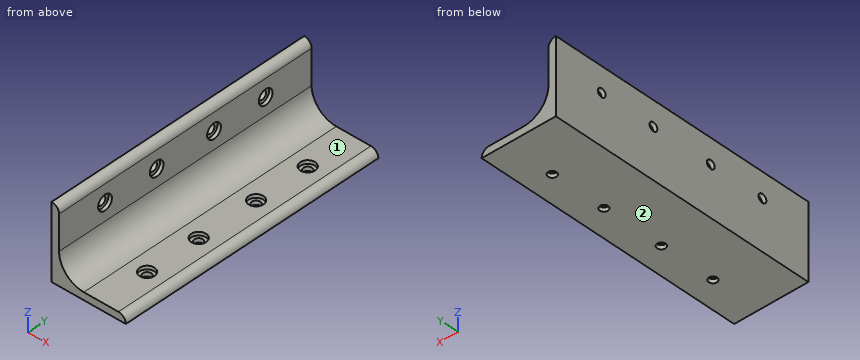
from build123d import *

# Parameters (mm, degrees)
BOSS_EXTRUDE1_DEPTH = 110
FILLET1_R           = 10
FILLET2_R           = 3
SKETCH2_R           = 1.7
CUT_EXTRUDE1_DEPTH  = 118.170815479
SKETCH3_R           = 1.7
CUT_EXTRUDE2_DEPTH  = 118.170815479
SKETCH4_R           = 3
CUT_EXTRUDE3_DEPTH  = 1.4
SKETCH5_R           = 3
CUT_EXTRUDE4_DEPTH  = 1.4


with BuildPart() as part:
    # Sketch1 → Boss-Extrude1 (new body)
    with BuildSketch(Plane(origin=(0, 0, 0), x_dir=(1, 0, 0), z_dir=(0, 1, 0))):
        Polygon((0, 0), (0, -30), (3, -30), (3, -3), (30, -3), (30, 0), align=None)
    extrude(amount=BOSS_EXTRUDE1_DEPTH)

    # Fillet1
    fillet1_edges = [part.edges().sort_by_distance(p)[0] for p in [
        (3, 55, 3),
    ]]
    fillet(fillet1_edges, radius=FILLET1_R)

    # Fillet2
    fillet2_edges = [part.edges().sort_by_distance(p)[0] for p in [
        (3, 55, 30),
        (30, 55, 3),
    ]]
    fillet(fillet2_edges, radius=FILLET2_R - 0.0001)  # a hair under: the kernel refuses the full size

    # Sketch2 → Cut-Extrude1 (cut, through all)
    with BuildSketch(Plane.XY.offset(3)):
        with Locations((20, 90)):
            Circle(SKETCH2_R)
        with Locations(Location((20, 67.5, 0), (0, 0, 180))):
            Circle(SKETCH2_R)
        with Locations((20, 42.5)):
            Circle(SKETCH2_R)
        with Locations(Location((20, 20, 0), (0, 0, 180))):
            Circle(SKETCH2_R)
    extrude(amount=-CUT_EXTRUDE1_DEPTH, mode=Mode.SUBTRACT)

    # Sketch3 → Cut-Extrude2 (cut, through all)
    with BuildSketch(Plane(origin=(3, 0, 0), x_dir=(0, 0, -1), z_dir=(1, 0, 0))):
        with Locations((-20, 90)):
            Circle(SKETCH3_R)
        with Locations(Location((-20, 67.5, 0), (0, 0, 180))):
            Circle(SKETCH3_R)
        with Locations((-20, 42.5)):
            Circle(SKETCH3_R)
        with Locations(Location((-20, 20, 0), (0, 0, 180))):
            Circle(SKETCH3_R)
    extrude(amount=-CUT_EXTRUDE2_DEPTH, mode=Mode.SUBTRACT)

    # Sketch4 → Cut-Extrude3 (cut)
    with BuildSketch(Plane.XY.offset(3)):
        with Locations((20, 90)):
            Circle(SKETCH4_R)
        with Locations(Location((20, 67.5, 0), (0, 0, 180))):
            Circle(SKETCH4_R)
        with Locations((20, 42.5)):
            Circle(SKETCH4_R)
        with Locations(Location((20, 20, 0), (0, 0, 180))):
            Circle(SKETCH4_R)
    extrude(amount=-CUT_EXTRUDE3_DEPTH, mode=Mode.SUBTRACT)

    # Sketch5 → Cut-Extrude4 (cut)
    with BuildSketch(Plane(origin=(3, 0, 0), x_dir=(0, 0, -1), z_dir=(1, 0, 0))):
        with Locations((-20, 90)):
            Circle(SKETCH5_R)
        with Locations(Location((-20, 67.5, 0), (0, 0, 180))):
            Circle(SKETCH5_R)
        with Locations((-20, 42.5)):
            Circle(SKETCH5_R)
        with Locations(Location((-20, 20, 0), (0, 0, 180))):
            Circle(SKETCH5_R)
    extrude(amount=-CUT_EXTRUDE4_DEPTH, mode=Mode.SUBTRACT)


solid = part.part
Model file for the job. Use its own axes, mm. Face numbers are marked on the shaded views. A direction names the side the tool comes from. Give positions to 0.01 mm unless a question says otherwise; leave off trailing zeros. One line per item, written item: value. Start each with the question number.
Q1. Probe probe 1 along Y at (x, z) = (20, 1.9); probe 2 along Y at (x, z) = (20, 0.8); probe 3 along Z at (x, y) = (14.75, 16). List the from-to ranges inside material, lowest first. Write a range as [from, to].
Q2. Saw through at A-A, the plane y = 90. State how many separate pieces and enclosed holes the cut face has, plus the area to 3 significant figures.
Q3. Drop flat-ended pins along their axis: pin 1 Ø4 at (x, y) = (22, 38) entering from +Z; pin 2 Ø10 at (x, y) = (11, 32.5) entering from +Z; pin 3 Ø3 at (x, y) = (19.5, 66.5) entering from +Z. Give the stop position or say it passes through.
Q4. 3-axis set-ups, long thin cutter, end or side, ignore diameter. For the marked faces 1 and 2: which of +Z, -Z, +X, -X, +Y, -Y reach the whole face in a straight line?
Output values:
1. probe 1: y = [0, 17], [23, 39.5], [45.5, 64.5], [70.5, 87], [93, 110]
1. probe 2: y = [0, 18.3], [21.7, 40.8], [44.2, 65.8], [69.2, 88.3], [91.7, 110]
1. probe 3: z = [0, 3]
2. separate pieces: 3
2. enclosed holes: 0
2. area: 161 mm²
3. pin 1: stops at z = 3
3. pin 2: stops at z = 5.86
3. pin 3: stops at z = 1.6
4. face 1: +Z, +X, +Y, -Y
4. face 2: -Z, +X, -X, +Y, -Y
